Verification items for the finished model (mm, model axes). A direction names the side the tool comes from. Coordinates: 2 decimals unless noted, no trailing zeros. Loops run counter-clockwise (first coordinate to the right, second up) from the corner with the lowest first, then second, coordinate; pieces in that order, holes last. Notation, with made-up numbers: (16.25, -13) - (20.25, -13) arc R15 ccw to (20.25, 1) - close; hole circle Ø4 at (52, 72.5). An arc over 180 degrees is marked (long way). One line per item, written item: value. Start each with the question number.
(1) Gauge pin test, flat ends, axial feed: P1, Ø3, axis at x = -7, z = 1.5, coming from the -Y side; P2, Ø1.1, axis at y = 4, z = -3, coming from the +X side; P3, Ø1.5, axis at x = -4.5, y = 11.5, coming from the -Z side; P4, Ø0.5, axis at y = 4, z = -3, coming from the -X side. Record the tip position at first contact, or that the pin passes through.
(2) Thickness scan on probe 1 along Z at (x, y) = (-8.5, 9.5); probe 2 along X at (y, z) = (2.25, -3.5); probe 3 along X at (y, z) = (3.5, 3.75). Record the ranges inside material, lowest first. Write a range as [from, to].
(3) Section check C-C (y = 6.75). Record the boundary of the cut face in (x, z).
(4) Section check A-A (z = -3). Record the boundary of the cut face in (x, y), plus the area to 3 significant figures.
(5) Section check D-D (z = -1). Record the boundary of the cut face in (x, y).
(6) Section check B-B (x = -27.5). Record the boundary of the cut face in (y, z), plus the area to 3 significant figures.
(7) Set-up check for faces 1 (the face through (-8, 4, -1)), 2 (the face through (-33, 4, -2.5)), 3 (the face through (-25.5, 4, -3)), 4 (the face through (-13, 4, -2.5)), 5 (the face through (-5.5, 4, -3)): record each of +Z, -Z, +X, -X, +Y, -Y from which the full face is reachable in a straight line by a thin tool's end or side.
(8) Draft check along Z on faces 6 (the face through (-20, 9, 3)), 7 (the face through (-41, 8, 3)), 8 (the face through (-20, 7, 5)), 9 (the face through (-13, 4, -5)). Enter one of: +Z half, -Z half, draft (parallel to the pull), parting line (faces both ways), or undercut.
```python
from build123d import *

# Parameters (mm, degrees)
SKETCH1_W           = 40
SKETCH1_H           = 15
BOSS_EXTRUDE1_DEPTH = 5
BOSS_EXTRUDE2_DEPTH = 7.5
SKETCH3_W           = 5
SKETCH3_H           = 15
BOSS_EXTRUDE3_DEPTH = 1
SKETCH4_W           = 40
SKETCH4_H           = 1
CUT_EXTRUDE1_DEPTH  = 12


with BuildPart() as part:
    # Sketch1 → Boss-Extrude1 (new body)
    with BuildSketch(Plane.XY):
        with Locations((-20, 7.5)):
            Rectangle(SKETCH1_W, SKETCH1_H)
    extrude(amount=BOSS_EXTRUDE1_DEPTH)

    # Sketch2 → Boss-Extrude2 (add)
    with BuildSketch(Plane.XZ):
        Polygon((-8, 0), (-12, 0), (-12, -2.5), (-14.5, -2.5), (-14.5, -3.5), (-12, -6), (-8, -6), (-5.5, -3.5), (-5.5, -2.5), (-8, -2.5), align=None)
    boss_extrude2 = extrude(amount=-BOSS_EXTRUDE2_DEPTH)

    # Mirror1: Boss-Extrude2 across plane
    add(boss_extrude2.mirror(Plane(origin=(-20, 0, 0), x_dir=(0, 0, 1), z_dir=(1, 0, 0))))

    # Sketch3 → Boss-Extrude3 (add)
    with BuildSketch(Plane(origin=(0, 0, 0), x_dir=(0, 0, -1), z_dir=(1, 0, 0))):
        with Locations((-2.5, 7.5)):
            Rectangle(SKETCH3_W, SKETCH3_H)
    boss_extrude3 = extrude(amount=BOSS_EXTRUDE3_DEPTH)

    # Mirror2: Boss-Extrude3 across plane
    add(boss_extrude3.mirror(Plane(origin=(-20, 0, 0), x_dir=(0, 0, 1), z_dir=(1, 0, 0))))

    # Sketch4 → Cut-Extrude1 (cut)
    with BuildSketch(Plane(origin=(0, 15, 0), x_dir=(1, 0, 0), z_dir=(0, 1, 0))):
        with Locations((-20, -3.5)):
            Rectangle(SKETCH4_W, SKETCH4_H)
    extrude(amount=-CUT_EXTRUDE1_DEPTH, mode=Mode.SUBTRACT)


solid = part.part
```
Responses:
1. P1: stops at y = 0
1. P2: stops at x = -5.5
1. P3: stops at z = 0
1. P4: stops at x = -34.5
2. probe 1: z = [0, 3], [4, 5]
2. probe 2: x = [-34.5, -25.5], [-14.5, -5.5]
2. probe 3: x = [-41, -40], [0, 1]
3. outline: (-41, 0) - (-32, 0) - (-32, -2.5) - (-34.5, -2.5) - (-34.5, -3.5) - (-32, -6) - (-28, -6) - (-25.5, -3.5) - (-25.5, -2.5) - (-28, -2.5) - (-28, 0) - (-12, 0) - (-12, -2.5) - (-14.5, -2.5) - (-14.5, -3.5) - (-12, -6) - (-8, -6) - (-5.5, -3.5) - (-5.5, -2.5) - (-8, -2.5) - (-8, 0) - (1, 0) - (1, 5) - (-41, 5) - close; hole (-40, 3) - (0, 3) - (0, 4) - (-40, 4) - close
4. outline: (-34.5, 0) - (-25.5, 0) - (-25.5, 7.5) - (-34.5, 7.5) - close; (-14.5, 0) - (-5.5, 0) - (-5.5, 7.5) - (-14.5, 7.5) - close
4. area: 135 mm²
5. outline: (-32, 0) - (-28, 0) - (-28, 7.5) - (-32, 7.5) - close; (-12, 0) - (-8, 0) - (-8, 7.5) - (-12, 7.5) - close
6. outline: (0, -5.5) - (7.5, -5.5) - (7.5, -2.5) - (0, -2.5) - close; (0, 0) - (15, 0) - (15, 3) - (3, 3) - (3, 4) - (15, 4) - (15, 5) - (0, 5) - close
6. area: 85.5 mm²
7. face 1: +X, +Y, -Y
7. face 2: -X, +Y, -Y
7. face 3: -Z, +Y, -Y
7. face 4: +Y, -Y
7. face 5: -Z, +X, +Y, -Y
8. face 6: undercut
8. face 7: draft
8. face 8: +Z half
8. face 9: -Z half
